Verification items for the finished model (mm, model axes). A direction names the side the tool comes from. Give positions to 0.01 mm unless a question says otherwise; leave off trailing zeros. Loops run counter-clockwise (first coordinate to the right, second up) from the corner with the lowest first, then second, coordinate; pieces in that order, holes last. Notation, with made-up numbers: (24.25, 53.5) - (72.25, 53.5) arc R14 ccw to (72.25, 67.5) - close; hole circle Ø10 at (36, 38.25). An arc over 180 degrees is marked (long way). One line per item, written item: value. Start each with the question number.
1. Sectioned sample at A-A (y = 7.25). Record the cut outline in (x, z), plus the area to 3 significant figures.
2. Access from +Z, -Z, +X, -X, +Y, -Y to the whole of each face (thin tool, end or side, straight path). Record for faces 5 (the flat face through (0, 8.205, -6)), 6 (the flat face through (3, 4.47, 4.17)), 7 (the flat face through (-1.343, 12.292, 1.993)).
3. Gauge pin test, flat ends, axial feed: pin 1 (3 mm diameter, centred on y = 2.5, z = -5, fed in from -X); pin 2 (4 mm diameter, centred on x = -5, z = 4, fed in from +Y); pin 3 (1.4 mm diameter, centred on x = 0.5, z = -7, fed in from +Y). Record the tip position at first contact, or that the pin passes through.
4. Mould release check, pull along X, two halves, no side actions. Record for faces 1 (the flat face through (-3.779, 5.15, -0.845)), 2 (the flat face through (0, 13.5, 0)), 3 (the flat face through (-0.27, 2.41, -3.56)), 4 (the flat face through (2.4, 3.2, -4.2)): pulls with the +X half, pulls with the -X half, needs draft (parallel to the pull), parting line crosses it, or undercut.
5. Sectioned sample at D-D (y = 4.5). Record the cut outline in (x, z), plus the area to 3 significant figures.
6. Sectioned sample at C-C (y = 10). Record the cut outline in (x, z), plus the area to 3 significant figures.
7. Sectioned sample at B-B (z = -5.5). Record the cut outline in (x, y).
8. Scan lines: L1, parallel to X at y = 8.5, z = 3.5; L2, parallel to Y at x = -4, z = -4; L3, parallel to X at y = 1, z = -3. Record each from-to range of solid material in increasing order. Write a range as [from, to].
from build123d import *
from OCP.BRepFilletAPI import BRepFilletAPI_MakeChamfer

# Parameters (mm, degrees)
SKETCH1_W           = 10
SKETCH1_H           = 10
BOSS_EXTRUDE1_DEPTH = 1.5
BOSS_EXTRUDE1_TAPER = 25
BOSS_EXTRUDE2_DEPTH = 12
CHAMFER1_SIZE       = 2
CHAMFER1_SIZE2      = 1.154700538
BOSS_EXTRUDE3_DEPTH = 10
CHAMFER2_SIZE       = 3
CHAMFER2_SIZE2      = 2.406716572
CHAMFER2_SIZE2_2    = 1.500380386
CHAMFER2_SIZE2_3    = 1.516874639
BOSS_EXTRUDE4_DEPTH = 8
BOSS_EXTRUDE5_DEPTH = 10
CHAMFER3_SIZE       = 4
CHAMFER3_SIZE2      = 2.031521954
CHAMFER3_SIZE2_2    = 2.008940765
CHAMFER3_SIZE2_3    = 2.098992436
CHAMFER3_SIZE2_4    = 2.518260147


with BuildPart() as part:
    # Sketch1 → Boss-Extrude1 (new body)
    with BuildSketch(Plane(origin=(0, 0, 0), x_dir=(1, 0, 0), z_dir=(0, 1, 0))):
        Rectangle(SKETCH1_W, SKETCH1_H)
    extrude(amount=BOSS_EXTRUDE1_DEPTH, taper=BOSS_EXTRUDE1_TAPER)

    # Sketch2 → Boss-Extrude2 (add)
    with BuildSketch(Plane(origin=(0, 1.5, 0), x_dir=(1, 0, 0), z_dir=(0, 1, 0))):
        Polygon((-2.812986954, -1.017959657), (-0.78305427, 4.14157821), (2.064873257, 0.914552857), (0.034940573, -4.24498501), align=None)
    extrude(amount=BOSS_EXTRUDE2_DEPTH)

    # Chamfer1: one chamfer whose edges measure the first distance from different faces: ONE call of the kernel's chamfer builder (chamfer() names one face for all edges)
    chamfer1_edges_1 = [part.edges().sort_by_distance(p)[0] for p in [
        (-1.389023191, 13.5, 2.631472333),
    ]]
    chamfer1_side_1 = [part.faces().sort_by_distance(p)[0] for p in [
        (-1.389023191, 7.5, 2.631472333),
    ]]
    chamfer1_edges_2 = [part.edges().sort_by_distance(p)[0] for p in [
        (1.049906915, 13.5, 1.665216077),
    ]]
    chamfer1_side_2 = [part.faces().sort_by_distance(p)[0] for p in [
        (1.049906915, 7.5, 1.665216077),
    ]]
    chamfer1_edges_3 = [part.edges().sort_by_distance(p)[0] for p in [
        (0.640909494, 13.5, -2.528065533),
    ]]
    chamfer1_side_3 = [part.faces().sort_by_distance(p)[0] for p in [
        (0.640909494, 7.5, -2.528065533),
    ]]
    chamfer1_edges_4 = [part.edges().sort_by_distance(p)[0] for p in [
        (-1.798020612, 13.5, -1.561809276),
    ]]
    chamfer1_side_4 = [part.faces().sort_by_distance(p)[0] for p in [
        (-1.798020612, 7.5, -1.561809276),
    ]]
    chamfer1 = BRepFilletAPI_MakeChamfer(part.part.solid().wrapped)
    for e in chamfer1_edges_1:
        chamfer1.Add(CHAMFER1_SIZE, CHAMFER1_SIZE2, e.wrapped, chamfer1_side_1[0].wrapped)  # the first distance lies on this face
    for e in chamfer1_edges_2:
        chamfer1.Add(CHAMFER1_SIZE, CHAMFER1_SIZE2, e.wrapped, chamfer1_side_2[0].wrapped)  # the first distance lies on this face
    for e in chamfer1_edges_3:
        chamfer1.Add(CHAMFER1_SIZE, CHAMFER1_SIZE2, e.wrapped, chamfer1_side_3[0].wrapped)  # the first distance lies on this face
    for e in chamfer1_edges_4:
        chamfer1.Add(CHAMFER1_SIZE, CHAMFER1_SIZE2, e.wrapped, chamfer1_side_4[0].wrapped)  # the first distance lies on this face
    add(Compound.cast(chamfer1.Shape()), mode=Mode.REPLACE)

    # Sketch4 → Boss-Extrude3 (add, along a direction that is not the sketch's normal)
    with BuildSketch(Plane(origin=(0, 1.5, 0), x_dir=(1, 0, 0), z_dir=(0, 1, 0))):
        Polygon((-3.685896684, -2.744355022), (-2.381707977, 1.767077084), (0.661288248, 0.315446351), (-0.642900459, -4.195985754), align=None)
    extrude(amount=BOSS_EXTRUDE3_DEPTH, dir=(-0.5520160266548657, 0.8281604089609962, 0.09710120156687128))

    # Chamfer2: one chamfer whose edges measure the first distance from different faces: ONE call of the kernel's chamfer builder (chamfer() names one face for all edges)
    chamfer2_edges_1 = [part.edges().sort_by_distance(p)[0] for p in [
        (-6.380370131, 9.78160409, -0.070249702),
    ]]
    chamfer2_side_1 = [part.faces().sort_by_distance(p)[0] for p in [
        (-7.032464485, 9.78160409, 2.185466351),
    ]]
    chamfer2_edges_2 = [part.edges().sort_by_distance(p)[0] for p in [
        (-8.553962597, 9.78160409, 1.459650985),
    ]]
    chamfer2_side_2 = [part.faces().sort_by_distance(p)[0] for p in [
        (-7.032464485, 9.78160409, 2.185466351),
    ]]
    chamfer2_edges_3 = [part.edges().sort_by_distance(p)[0] for p in [
        (-7.684558838, 9.78160409, 4.441182404),
    ]]
    chamfer2_side_3 = [part.faces().sort_by_distance(p)[0] for p in [
        (-4.924478705, 5.640802045, 3.955676396),
    ]]
    chamfer2 = BRepFilletAPI_MakeChamfer(part.part.solid().wrapped)
    for e in chamfer2_edges_1:
        chamfer2.Add(CHAMFER2_SIZE, CHAMFER2_SIZE2, e.wrapped, chamfer2_side_1[0].wrapped)  # the first distance lies on this face
    for e in chamfer2_edges_2:
        chamfer2.Add(CHAMFER2_SIZE, CHAMFER2_SIZE2_2, e.wrapped, chamfer2_side_2[0].wrapped)  # the first distance lies on this face
    for e in chamfer2_edges_3:
        chamfer2.Add(CHAMFER2_SIZE, CHAMFER2_SIZE2_3, e.wrapped, chamfer2_side_3[0].wrapped)  # the first distance lies on this face
    add(Compound.cast(chamfer2.Shape()), mode=Mode.REPLACE)

    # Sketch5 → Boss-Extrude4 (add, along a direction that is not the sketch's normal)
    with BuildSketch(Plane(origin=(0, 1.5, 0), x_dir=(1, 0, 0), z_dir=(0, 1, 0))):
        Polygon((-0.799065943, 0.680702687), (0.288664987, -2.936597885), (4.019801987, -2.756774896), (2.932071057, 0.860525676), align=None)
    extrude(amount=BOSS_EXTRUDE4_DEPTH, dir=(0.12852896278760917, 0.6705109361257466, 0.7306814560809083))

    # Sketch6 → Boss-Extrude5 (add, along a direction that is not the sketch's normal)
    with BuildSketch(Plane(origin=(0, 1.5, 0), x_dir=(1, 0, 0), z_dir=(0, 1, 0))):
        Polygon((-1.600069282, 0), (1.180756558, -2.337369015), (4.1003801, 1.192394032), (1.31955426, 3.529763047), align=None)
    extrude(amount=BOSS_EXTRUDE5_DEPTH, dir=(-0.12852896278760925, 0.6705109361257466, -0.7306814560809083))

    # Chamfer3: one chamfer whose edges measure the first distance from different faces: ONE call of the kernel's chamfer builder (chamfer() names one face for all edges)
    chamfer3_edges_1 = [part.edges().sort_by_distance(p)[0] for p in [
        (-1.425547139, 8.205109361, -9.071696084),
    ]]
    chamfer3_side_1 = [part.faces().sort_by_distance(p)[0] for p in [
        (-0.77862694, 5.370569751, -6.108006882),
    ]]
    chamfer3_edges_2 = [part.edges().sort_by_distance(p)[0] for p in [
        (1.424677552, 8.205109361, -9.6678931),
    ]]
    chamfer3_side_2 = [part.faces().sort_by_distance(p)[0] for p in [
        (2.067322366, 4.852554681, -6.01448582),
    ]]
    chamfer3_edges_3 = [part.edges().sort_by_distance(p)[0] for p in [
        (3.182465189, 6.864087489, 8.692138039),
    ]]
    chamfer3_side_3 = [part.faces().sort_by_distance(p)[0] for p in [
        (2.674699398, 4.189172634, 5.776940656),
    ]]
    chamfer3_edges_4 = [part.edges().sort_by_distance(p)[0] for p in [
        (4.504168224, 6.864087489, 6.793576259),
    ]]
    chamfer3_side_4 = [part.faces().sort_by_distance(p)[0] for p in [
        (3.998071432, 4.203478125, 3.907212333),
    ]]
    chamfer3 = BRepFilletAPI_MakeChamfer(part.part.solid().wrapped)
    for e in chamfer3_edges_1:
        chamfer3.Add(CHAMFER3_SIZE, CHAMFER3_SIZE2, e.wrapped, chamfer3_side_1[0].wrapped)  # the first distance lies on this face
    for e in chamfer3_edges_2:
        chamfer3.Add(CHAMFER3_SIZE, CHAMFER3_SIZE2_2, e.wrapped, chamfer3_side_2[0].wrapped)  # the first distance lies on this face
    for e in chamfer3_edges_3:
        chamfer3.Add(CHAMFER3_SIZE, CHAMFER3_SIZE2_3, e.wrapped, chamfer3_side_3[0].wrapped)  # the first distance lies on this face
    for e in chamfer3_edges_4:
        chamfer3.Add(CHAMFER3_SIZE, CHAMFER3_SIZE2_4, e.wrapped, chamfer3_side_4[0].wrapped)  # the first distance lies on this face
    add(Compound.cast(chamfer3.Shape()), mode=Mode.REPLACE)


solid = part.part
Results are:
1. outline: (-7.48, 3.28) - (-6.21, -1.09) - (-3.17, 0.36) - (-4.44, 4.73) - close; (-2.81, 1.02) - (-0.78, -4.14) - (2.06, -0.91) - (0.03, 4.24) - close; (-1.63, -5.37) - (0.38, -7.8) - (2.09, -6.36) - (0.08, -3.93) - close
1. area: 43.5 mm^2
2. face 5: -Z, +X, -X, +Y
2. face 6: +X, +Y
2. face 7: +Z, -X, +Y
3. pin 1: stops at x = -4.49
3. pin 2: stops at y = 9.78
3. pin 3: stops at y = 8.21
4. face 1: undercut
4. face 2: needs draft
4. face 3: undercut
4. face 4: pulls with the +X half
5. outline: (-5.69, 3.1) - (-4.38, -1.42) - (-2.25, -0.4) - (-1.39, -2.61) - (-2.18, -3.27) - (0.74, -6.8) - (3.53, -4.46) - (1.3, -1.78) - (2.06, -0.91) - (0.7, 2.54) - (2.46, 2.46) - (3.47, 5.82) - (0.79, 5.95) - (0.17, 3.9) - (0.03, 4.24) - (-1.92, 2.03) - (-2.64, 4.55) - close
5. area: 56.3 mm^2
6. outline: (-2.81, 1.02) - (-0.78, -4.14) - (2.06, -0.91) - (0.03, 4.24) - close
6. area: 21.2 mm^2
7. outline: (-1.57, 7.45) - (-1.04, 5.15) - (0.97, 3.31) - (2.78, 4.94) - (2.91, 5.85) - (0.33, 8.21) - (-0.74, 8.21) - close
8. L1: x = [-6.58, -4.87], [-0.62, 0.33]
8. L2: y = [0, 1.5]
8. L3: x = [-4.53, 4.53]
